Source: CAD feature listing. Evaluate the final solid. Frame: model axes, mm. Give positions to 0.01 mm unless a question says otherwise; leave off trailing zeros. Order: outer loops, then holes, each group sorted by start corner. A loop starts at its lowest first (then second) coordinate and runs counter-clockwise, first axis right, second up. Notation, with made-up numbers: M -36,68.5 L 13,68.5 A33 cw 13,99.5 Z; hole C 41,-6 d6. An arc over 180 degrees is marked long. Use CSV: the item, a comma, the result in double quotes. Start each with the question number.
1. Section query B-B, the plane x = 183. Return the cut outline in (y, z), plus the area to 3 significant figures.
2. Section query C-C, the plane z = -64.5. Return the cut outline in (x, y).
3. Pin query (flat end, axial travel): P1, Ø1.5, axis at y = 1, z = 147, coming from the -X side; P2, Ø1.5, axis at y = 1, z = 90.5, coming from the +X side; P3, Ø0.9, axis at x = 319.5, y = 1, coming from the +Z side. Return the tip coordinate at first contact, or that it passes through.
4. Line query: line 1 along X through (y, z) = (2.8, 102.5); line 2 along X through (y, z) = (1.65, -34); line 3 along Z through (x, y) = (287.5, 2.1). Output: solid intervals per line, ascending. Write a range as [from, to].
5. Section query A-A, the plane y = 0.95. Return the cut outline in (x, z), plus the area to 3 significant figures.
from build123d import *

# Parameters (mm, degrees)
CROQUIS1_W              = 250
CROQUIS1_H              = 250
SALIENTE_EXTRUIR1_DEPTH = 3
CROQUIS2_W              = 250
CROQUIS2_H              = 3
SALIENTE_EXTRUIR2_DEPTH = 3
CROQUIS3_W              = 220
CROQUIS3_H              = 99.34
SALIENTE_EXTRUIR4_DEPTH = 3
CROQUIS4_W              = 41
CROQUIS4_H              = 52
CORTAR_EXTRUIR1_DEPTH   = 3
CORTAR_EXTRUIR2_DEPTH   = 3
CROQUIS6_W              = 339
CROQUIS6_H              = 30
SALIENTE_EXTRUIR5_DEPTH = 3
CORTAR_EXTRUIR3_DEPTH   = 3
CROQUIS8_W              = 1
CROQUIS8_H              = 44
SALIENTE_EXTRUIR6_DEPTH = 3
SALIENTE_EXTRUIR7_DEPTH = 3
CROQUIS10_W             = 41
CROQUIS10_H             = 6
SALIENTE_EXTRUIR9_DEPTH = 3
CROQUIS11_W             = 40
CROQUIS11_H             = 1
CORTAR_EXTRUIR4_DEPTH   = 3


with BuildPart() as part:
    # Croquis1 → Saliente-Extruir1 (new body)
    with BuildSketch(Plane(origin=(0, 0, 0), x_dir=(1, 0, 0), z_dir=(0, 1, 0))):
        Rectangle(CROQUIS1_W, CROQUIS1_H)
    extrude(amount=SALIENTE_EXTRUIR1_DEPTH)

    # Croquis2 → Saliente-Extruir2 (add)
    with BuildSketch(Plane(origin=(0, 3, 0), x_dir=(1, 0, 0), z_dir=(0, 1, 0))):
        with Locations((0, 126.5)):
            Rectangle(CROQUIS2_W, CROQUIS2_H)
    extrude(amount=-SALIENTE_EXTRUIR2_DEPTH)

    # Croquis3 → Saliente-Extruir4 (add)
    with BuildSketch(Plane(origin=(0, 3, 0), x_dir=(1, 0, 0), z_dir=(0, 1, 0))):
        with Locations((235, -75.33)):
            Rectangle(CROQUIS3_W, CROQUIS3_H)
    extrude(amount=-SALIENTE_EXTRUIR4_DEPTH)

    # Croquis4 → Cortar-Extruir1 (cut)
    with BuildSketch(Plane(origin=(0, 3, 0), x_dir=(1, 0, 0), z_dir=(0, 1, 0))):
        with Locations((-104.5, -99)):
            Rectangle(CROQUIS4_W, CROQUIS4_H)
    extrude(amount=-CORTAR_EXTRUIR1_DEPTH, mode=Mode.SUBTRACT)

    # Croquis5 → Cortar-Extruir2 (cut)
    with BuildSketch(Plane(origin=(0, 3, 0), x_dir=(1, 0, 0), z_dir=(0, 1, 0))):
        with BuildLine():
            Line((-84, -116), (-84, -125))
            Line((-84, -125), (-75, -125))
            ThreePointArc((-75, -125), (-81.363961031, -122.363961031), (-84, -116))
        make_face()
    extrude(amount=-CORTAR_EXTRUIR2_DEPTH, mode=Mode.SUBTRACT)

    # Croquis6 → Saliente-Extruir5 (add)
    with BuildSketch(Plane(origin=(0, 3, 0), x_dir=(1, 0, 0), z_dir=(0, 1, 0))):
        with Locations((110.5, -140)):
            Rectangle(CROQUIS6_W, CROQUIS6_H)
    extrude(amount=-SALIENTE_EXTRUIR5_DEPTH)

    # Croquis7 → Cortar-Extruir3 (cut)
    with BuildSketch(Plane(origin=(0, 3, 0), x_dir=(1, 0, 0), z_dir=(0, 1, 0))):
        with BuildLine():
            Line((345, -72), (304, -72))
            Line((304, -72), (304, -116))
            ThreePointArc((304, -116), (301.363961031, -122.363961031), (295, -125))
            Line((295, -125), (345, -125))
            Line((345, -125), (345, -72))
        make_face()
    extrude(amount=-CORTAR_EXTRUIR3_DEPTH, mode=Mode.SUBTRACT)

    # Croquis8 → Saliente-Extruir6 (add)
    with BuildSketch(Plane(origin=(0, 3, 0), x_dir=(1, 0, 0), z_dir=(0, 1, 0))):
        with Locations((304.5, -94)):
            Rectangle(CROQUIS8_W, CROQUIS8_H)
    extrude(amount=-SALIENTE_EXTRUIR6_DEPTH)

    # Croquis9 → Saliente-Extruir7 (add)
    with BuildSketch(Plane(origin=(0, 3, 0), x_dir=(1, 0, 0), z_dir=(0, 1, 0))):
        with BuildLine():
            Line((295, -125), (296, -125))
            ThreePointArc((296, -125), (302.363961031, -122.363961031), (305, -116))
            Line((305, -116), (304, -116))
            Line((304, -116), (295, -125))
        make_face()
    extrude(amount=-SALIENTE_EXTRUIR7_DEPTH)

    # Croquis10 → Saliente-Extruir9 (add)
    with BuildSketch(Plane(origin=(0, 3, 0), x_dir=(1, 0, 0), z_dir=(0, 1, 0))):
        with Locations((-104.5, -76)):
            Rectangle(CROQUIS10_W, CROQUIS10_H)
    extrude(amount=-SALIENTE_EXTRUIR9_DEPTH)

    # Croquis11 → Cortar-Extruir4 (cut)
    with BuildSketch(Plane(origin=(0, 3, 0), x_dir=(1, 0, 0), z_dir=(0, 1, 0))):
        with Locations((325, -71.5)):
            Rectangle(CROQUIS11_W, CROQUIS11_H)
    extrude(amount=-CORTAR_EXTRUIR4_DEPTH, mode=Mode.SUBTRACT)


solid = part.part
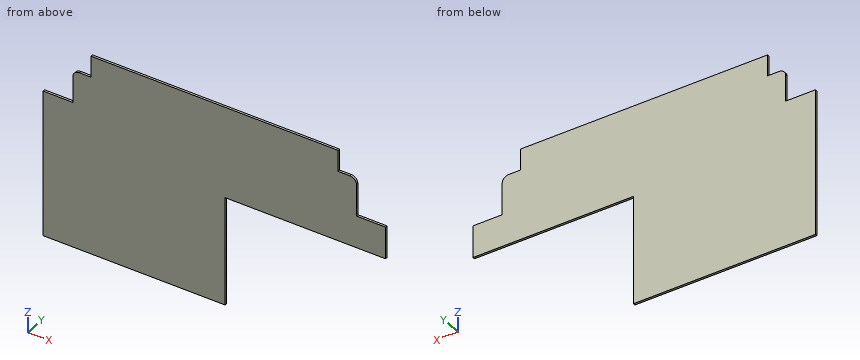
Result set:
1,outline,"M 0,25.66 L 3,25.66 L 3,155 L 0,155 Z"
1,area,"388 mm2"
2,outline,"M -125,0 L 125,0 L 125,3 L -125,3 Z"
3,P1,"x = -59"
3,P2,"x = 305"
3,P3,"z = 71"
4,line 1,"[-84, 305]"
4,line 2,"[-125, 125]"
4,line 3,"[25.66, 125]"
5,outline,"M -125,-128 L 125,-128 L 125,25.66 L 345,25.66 L 345,71 L 305,71 L 305,116 A9 ccw 296,125 L 280,125 L 280,155 L -59,155 L -59,125 L -75,125 A9 ccw -84,116 L -84,79 L -125,79 Z"
5,area,"91,200 mm2"
